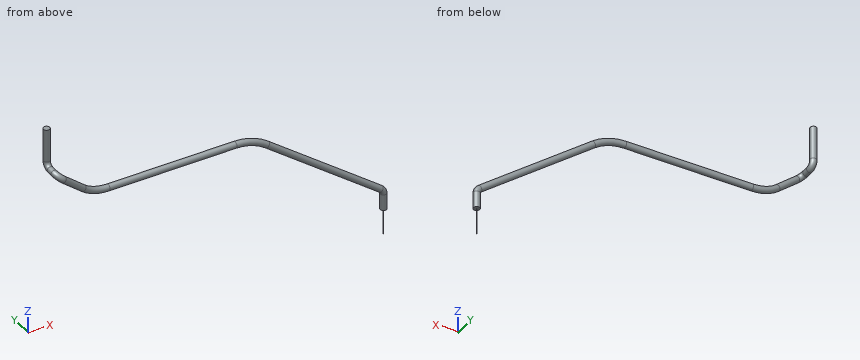
from build123d import *

# Parameters (mm, degrees)
SKETCH1_R           = 1.5
SKETCH2_R           = 0.125
BOSS_EXTRUDE1_DEPTH = 12.5


with BuildPart() as part:
    # Base-Sweep: sweep along a curve in space
    with BuildLine() as base_sweep_path:
        Line((60.65, -0.65, 0), (60.65, -0.65, 7.75208786))
        ThreePointArc((59.424167714, -0.560464146, 10.173638084), (60.325999238, -0.626334703, 9.109897397), (60.65, -0.65, 7.75208786))
        Line((59.424167714, -0.560464146, 10.173638084), (7.590881524, 3.225484065, 48.180781395))
        ThreePointArc((-7.239671238, 3.708602428, 53.030807816), (0.565798877, 3.584726574, 51.787217816), (7.590881524, 3.225484065, 48.180781395))
        Line((-7.239671238, 3.708602428, 53.030807816), (-67.575239414, 3.708602428, 53.030807816))
        ThreePointArc((-80.211652793, 2.635461889, 57.72083447), (-74.335914745, 3.431241001, 54.242981282), (-67.575239414, 3.708602428, 53.030807816))
        Line((-80.211652793, 2.635461889, 57.72083447), (-90.877343373, 0.516767824, 66.980322185))
        ThreePointArc((-93.478797639, 3.483575243, 69.238791399), (-92.69169695, 1.210351005, 68.555464885), (-90.877343373, 0.516767824, 66.980322185))
        Line((-93.478797639, 3.483575243, 69.238791399), (-93.478797639, 6.5, 69.238791399))
        ThreePointArc((-93.478797639, 9.5, 72.238791399), (-93.478797639, 8.621320344, 70.117471055), (-93.478797639, 6.5, 69.238791399))
        Line((-93.478797639, 9.5, 72.238791399), (-93.478797639, 9.5, 88.091291399))
    # Sketch1 → Base-Sweep (sweep)
    with BuildSketch(Plane.XY):
        with Locations((60.65, -0.65)):
            Circle(SKETCH1_R)
    sweep(path=base_sweep_path.line)

    # Sketch2 → Boss-Extrude1 (add)
    with BuildSketch(Plane(origin=(0, 0, 0), x_dir=(-1, 0, 0), z_dir=(0, 0, -1))):
        with Locations(Location((-60.65, -0.65, 0), (0, 0, 180))):
            Circle(SKETCH2_R)
    extrude(amount=BOSS_EXTRUDE1_DEPTH)


solid = part.part
Work out the finished part from the listing and answer in its coordinate system (mm). Coordinates: 2 decimals unless noted, no trailing zeros. Loops run counter-clockwise (first coordinate to the right, second up) from the corner with the lowest first, then second, coordinate; pieces in that order, holes last. Notation, with made-up numbers: (89, 19) -> (114, 19) arc R7 ccw to (114, 29) -> close; hole circle Ø3 at (77, 16.5). An arc over 180 degrees is marked (long way). Write each question's results on one line, items separated by ' | '. Start each with the question number.
1) Flat-ended cylindrical pins translate along their axes: P1, Ø1, axis at x = -55, y = 3, coming from the -Z side; P2, Ø3, axis at y = 4.5, z = 72, coming from the -X side. Find the tip coordinate at first contact, or state that the pin passes through.
2) Consider line 1 along Z through (x, y) = (-55, 3.75); line 2 along X through (y, z) = (7, 69); line 3 along Z through (x, y) = (12, 3.5). Determine where each line is inside the solid, lowest interval first.
3) Find section A-A on z = 2. Determine the outline of the cut face in (x, y).
Response values:
1) P1: stops at z = 51.55 | P2: stops at x = -94.29
2) line 1: z = 51.53 to 54.53 | line 2: x = -94.95 to -92 | line 3: z = 43.27 to 46.69
3) outline: circle Ø3 at (60.65, -0.65)
